Autodesk Inventor part; units mm, degrees
ref_plane "Work Plane1" through (-35.3023, 0, 0) normal (0, -0.866, -0.5) x (1, 0, 0)
ref_plane "YZ Plane" through (0, 0, 0) normal (1, 0, 0) x (0, 1, 0)
ref_plane "XZ Plane" through (0, 0, 0) normal (0, 1, 0) x (-1, 0, 0)
sketch "Sketch1" plane through (0, 0, 0) normal (1, 0, 0) x (0, 1, 0)
  line L0 (-19.2401, 0) -> (-9.62, 16.6624)
  line L1 (-9.62, 16.6624) -> (9.62, 16.6624)
  line L2 (9.62, 16.6624) -> (19.2401, 0)
  line L3 (19.2401, 0) -> (9.62, -16.6624)
  line L4 (9.62, -16.6624) -> (-9.62, -16.6624)
  line L5 (-9.62, -16.6624) -> (-19.2401, 0)
  point P0 (0, 0)
  point P1 (0, 0)
  dimension "d0" = 38.4802
extrude "Body" add sketch "Sketch1" along normal blind 19.05
sketch "Sketch2" plane through (0, 0, 0) normal (0, 0, 1) x (1, 0, 0)
  line L0 (0, 9.62) -> (0, 19.2401)
  line L1 (0, 19.2401) -> (19.05, 19.2401)
  line L2 (19.05, 9.62) -> (19.05, 19.2401)
  line L3 (-3.81, 0) -> (22.86, 0)
  line L4 (1.4882, 19.2401) -> (0, 16.6624)
  line L5 (17.5618, 19.2401) -> (19.05, 16.6624)
  dimension "d3" = 30
  dimension "d4" = 30
  dimension "d5" = 33.3248
  dimension "d6" = 33.3248
revolve "Chamfer1" cut sketch "Sketch2" angle 360 about axis through (-10, 0, 0) along (1, 0, 0)
sketch "Sketch3" plane through (19.05, 0, 0) normal (1, 0, 0) x (0, 0, -1)
  arc A0 (-8.3312, -14.4301) -> (8.3312, -14.4301) centre (0, 0) ccw
hole "Thread" at (19.05, 0, 0) direction (-1, 0, 0) diameter 19.177 end through all
chamfer "Chamfer2" distance 1.5276 angle 30 1 edges at (19.05, 0, 9.5885) measured on face at (19.05, 14.2203, -0.3853)
chamfer "Chamfer3" distance 1.5276 angle 30 1 edges at (0, 0, 9.5885) measured on face at (0, 14.2203, -0.3853)
ref_plane "Work Plane1" through (-35.3023, 0, 0) normal (0, -0.866, -0.5) x (1, 0, 0)
equation "\"d0\" = 1.1547 * SW"
equation "\"d1\" = KOH"
equation "\"d3\" = ANG1"
equation "\"d4\" = ANG2"
equation "\"d5\" = SW0"
equation "\"d6\" = SW01"
equation "\"d8\" = -0.5 * GD1 + 0.5 * NND"
equation "\"d40\" = -0.5 * GD1 + 0.5 * NND"
equation "\"d10\" = -0.5 * GD1 + 0.5 * NND"
equation "\"d41\" = -0.5 * GD1 + 0.5 * NND"
equation "\"ANG1\" = 30deg"
equation "\"ANG2\" = 30deg"
equation "\"NND\" = 22.225"
equation "\"KOH\" = 19.05"
equation "\"SW\" = 33.3248"
equation "\"SW0\" = SW"
equation "\"SW01\" = SW"
equation "\"THREADDIA\" = 22.225"
equation "\"TOA\" = 30deg"
equation "\"E0\" = 1.155 * SW"
properties part number "ANSI B18.2.2 - 7/8 - 9" material "Steel, Mild"
Input: part model. Units: mm. Frame: model coordinates. Coordinates: 2 decimals unless noted, no trailing zeros. Loops run counter-clockwise (first coordinate to the right, second up) from the corner with the lowest first, then second, coordinate; pieces in that order, holes last. Notation, with made-up numbers: (44.25, -38.75) -> (79.25, -38.75) arc R30 cw to (79.25, -0.75) -> close; hole circle Ø7 at (42, 41.5). An arc over 180 degrees is marked (long way). One line per item, written item: value.
(1) Cut plane A-A (x = 15.75). Output: boundary loops of the cut face in (y, z), then the cut area to 3 significant figures.
Answer below:
outline: (-19.24, 0) -> (-9.62, -16.66) -> (9.62, -16.66) -> (19.24, 0) -> (9.62, 16.66) -> (-9.62, 16.66) -> close; hole circle Ø19.18 at (0, 0)
area: 673 mm2
(2) Ray query, line 1 along Y through (x, z) = (14.5, 0); line 2 along Z through (x, y) = (5, 0); line 3 along Y through (x, z) = (17.5, -2). Return the intervals inside material, ascending.
Answer below:
line 1: y = -19.24 to -9.59, 9.59 to 19.24
line 2: z = -16.66 to -9.59, 9.59 to 16.66
line 3: y = -18.09 to -9.38, 9.38 to 18.09
(3) Draft query along Z for faces 1 (the face through (0.362, 17.289, -0.042)), 2 (the face through (18.69, -8.68, 14.95)), 3 (the face through (0.8, 9.5, 2.1)). Return one class per face: pulls with the +Z half, pulls with the -Z half, needs draft (parallel to the pull), parting line crosses it, or undercut.
Answer below:
face 1: parting line crosses it
face 2: pulls with the +Z half
face 3: undercut
